The listing builds one solid part. Answer for the finished solid, in the listing's coordinates (mm). Face numbers are marked on the shaded views. A direction names the side the tool comes from. Round coordinates to 2 decimals unless told otherwise and drop trailing zeros. Order: outer loops, then holes, each group sorted by start corner. A loop starts at its lowest first (then second) coordinate and runs counter-clockwise, first axis right, second up. Notation, with made-up numbers: (-19, 83) -> (22, 83) arc R28 ccw to (22, 102) -> close; hole circle Ø7 at (72.25, 26). An arc over 180 degrees is marked (long way). Answer in a Markdown table with one row per item. Add a question column.
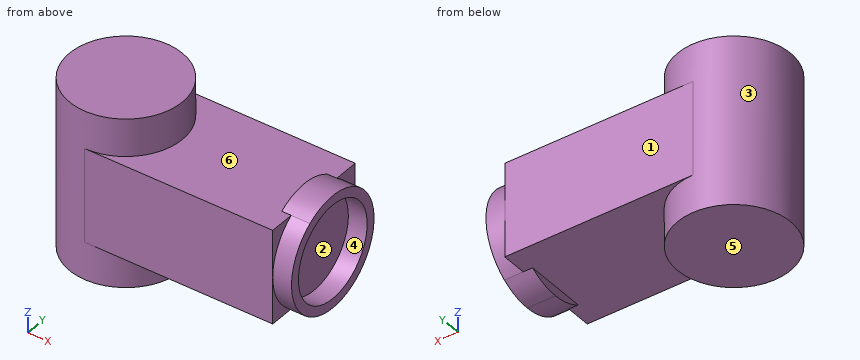
```python
from build123d import *

# Parameters (mm, degrees)
SKETCH3_W                = 100
SKETCH3_H                = 60
BOSS_EXTRUDE3_DEPTH      = 25
SKETCH4_R                = 30
BOSS_EXTRUDE5_DEPTH      = 45
BOSS_EXTRUDE9_DEPTH      = 10
BOSS_EXTRUDE9_DEPTH_BACK = 5


with BuildPart() as part:
    # Sketch3 → Boss-Extrude3 (new, symmetric)
    with BuildSketch(Plane.XY):
        Rectangle(SKETCH3_W, SKETCH3_H)
    extrude(amount=BOSS_EXTRUDE3_DEPTH, both=True)

    # Sketch4 → Boss-Extrude5 (add, symmetric)
    with BuildSketch(Plane.XY):
        with Locations((-50, 0)):
            Circle(SKETCH4_R)
    extrude(amount=BOSS_EXTRUDE5_DEPTH, both=True)

    # Sketch5 → Boss-Extrude9 (add, two sides: drawn at the far end of the back side and taken through both)
    with BuildSketch(Plane(origin=(50, 0, 0), x_dir=(0, 0, -1), z_dir=(1, 0, 0)).offset(-BOSS_EXTRUDE9_DEPTH_BACK)):
        with BuildLine():
            Line((-25, 2.6e-08), (-25, 16.583123952))
            ThreePointArc((-25, 16.583123952), (-30, 0), (-25, -16.583123952))
            Line((-25, -16.583123952), (-25, 2.6e-08))
        make_face()
        with BuildLine():
            Line((25, 0), (25, 16.583123952))
            ThreePointArc((25, 16.583123952), (0, 30), (-25, 16.583123952))
            Line((-25, 16.583123952), (-25, 2.6e-08))
            ThreePointArc((-25, 2.6e-08), (1.3e-08, 25), (25, 0))
        make_face()
        with BuildLine():
            ThreePointArc((-25, -16.583123952), (0, -30), (25, -16.583123952))
            Line((25, -16.583123952), (25, 0))
            ThreePointArc((25, 0), (-1.3e-08, -25), (-25, 2.6e-08))
            Line((-25, 2.6e-08), (-25, -16.583123952))
        make_face()
        with BuildLine():
            ThreePointArc((25, -16.583123952), (28.722813233, -8.660254038), (30, 0))
            ThreePointArc((30, 0), (28.722813233, 8.660254038), (25, 16.583123952))
            Line((25, 16.583123952), (25, 0))
            Line((25, 0), (25, -16.583123952))
        make_face()
    extrude(amount=BOSS_EXTRUDE9_DEPTH + BOSS_EXTRUDE9_DEPTH_BACK)


solid = part.part
```
1. The part is cut by section C-C (y = 13). Give the vertices of the cut face in (x, z).
2. Straight lines are drawn through the part: line 1 along Y through (x, z) = (53.75, 0); line 2 along Z through (x, y) = (-4, -13); line 3 along Z through (x, y) = (53, 16.5). For each, find the intervals that lie inside material, in ascending order.
3. The part is cut by section A-A (y = 4.5). Give the vertices of the cut face in (x, z), then the cut area to 3 significant figures.
4. The mould has two halves that part along Z. Classify the marked faces 4, 5 and 6: released by +Z, released by -Z, zero draft, split by the parting line, or undercut.
5. The part is cut by section B-B (z = 35). Give the vertices of the cut face in (x, y), then the cut area to 3 significant figures.
6. Each of these flat-tipped pins is pushed along its axis until it touches: pin 1 (2.5 mm diameter, centred on y = -5.5, z = -26.5, fed in from -X); pin 2 (3 mm diameter, centred on x = -15, y = -4, fed in from -Z); pin 3 (1.5 mm diameter, centred on y = -1.5, z = 28.5, fed in from -X). Where does it stop, or does it pass through?
7. The part is cut by section D-D (z = -11). Give the vertices of the cut face in (x, y), then the cut area to 3 significant figures.
8. For the marked faces 1, 2 and 3, determine the directions among +Z, -Z, +X, -X, +Y, -Y from which every point of the face is accessible in a straight line to the end or side of a thin tool.
Report:
| question | item | result |
|---|---|---|
| 1 | outline | (-77.04, -45) -> (-22.96, -45) -> (-22.96, -25) -> (45, -25) -> (45, -27.04) -> (60, -27.04) -> (60, -21.35) -> (50, -21.35) -> (50, 21.35) -> (60, 21.35) -> (60, 27.04) -> (45, 27.04) -> (45, 25) -> (-22.96, 25) -> (-22.96, 45) -> (-77.04, 45) -> close |
| 2 | line 1 | y = -30 to -25, 25 to 30 |
| 2 | line 2 | z = -25 to 25 |
| 2 | line 3 | z = -25.05 to -18.78, 18.78 to 25.05 |
| 3 | outline | (-79.66, -45) -> (-20.34, -45) -> (-20.34, -25) -> (45, -25) -> (45, -29.66) -> (60, -29.66) -> (60, -24.59) -> (50, -24.59) -> (50, 24.59) -> (60, 24.59) -> (60, 29.66) -> (45, 29.66) -> (45, 25) -> (-20.34, 25) -> (-20.34, 45) -> (-79.66, 45) -> close |
| 3 | area | 9,000 mm^2 |
| 4 | face 4 | undercut |
| 4 | face 5 | released by -Z |
| 4 | face 6 | released by +Z |
| 5 | outline | circle Ø60 at (-50, 0) |
| 5 | area | 2,830 mm^2 |
| 6 | pin 1 | stops at x = -79.7 |
| 6 | pin 2 | stops at z = -25 |
| 6 | pin 3 | stops at x = -79.99 |
| 7 | outline | (-50, -30) -> (50, -30) -> (50, -27.91) -> (60, -27.91) -> (60, -22.45) -> (50, -22.45) -> (50, 22.45) -> (60, 22.45) -> (60, 27.91) -> (50, 27.91) -> (50, 30) -> (-50, 30) arc R30 ccw to start |
| 7 | area | 7,520 mm^2 |
| 8 | face 1 | +Z, -Z, +X, -X, +Y |
| 8 | face 2 | +X |
| 8 | face 3 | none |
